Verification items for this drawing (mm, ordinates from the low corner). A direction names the side the tool comes from. Round coordinates to 2 decimals unless told otherwise and drop trailing zeros. Loops run counter-clockwise (first coordinate to the right, second up) from the corner with the lowest first, then second, coordinate; pieces in that order, holes last. Notation, with made-up numbers: M -16.75,20 L 31.25,20 A38 ccw 31.25,59 Z; hole C 84.5,38.25 d4. An arc over 180 degrees is marked long. Write item = value, one per line. Start each with the question number.
(1) Cross-section at D-D on x = 5.1. Record the boundary of the cut face in (y, z), plus the area to 3 significant figures.
(2) Cross-section at C-C on y = 11.25. Record the boundary of the cut face in (x, z), plus the area to 3 significant figures.
(3) Scan lines: L1, parallel to Y at x = 4.8, z = 4.45; L2, parallel to Z at x = 2.85, y = 4.5; L3, parallel to X at y = 5.25, z = 3.9. Record each from-to range of solid material in increasing order. Write a range as from..to.
(4) Go/stop test with flat-tipped pins: P1, Ø1.5, axis at x = 4.5, z = 1.5, coming from the -Y side; P2, Ø1.5, axis at y = 5, z = 5, coming from the -X side (1 decimal); P3, Ø3.5, axis at y = 5, z = 3, coming from the +X side. Record where each tip stops, or that it passes through.
(5) Cross-section at B-B on z = 2. Record the boundary of the cut face in (x, y), plus the area to 3 significant figures.
(6) Set-up check for the marked faces 1, 2, 3, 4 and 5: record each of +Z, -Z, +X, -X, +Y, -Y from which the full face is reachable in a straight line by a thin tool's end or side.
(7) Cross-section at A-A on x = 0.45. Record the boundary of the cut face in (y, z).
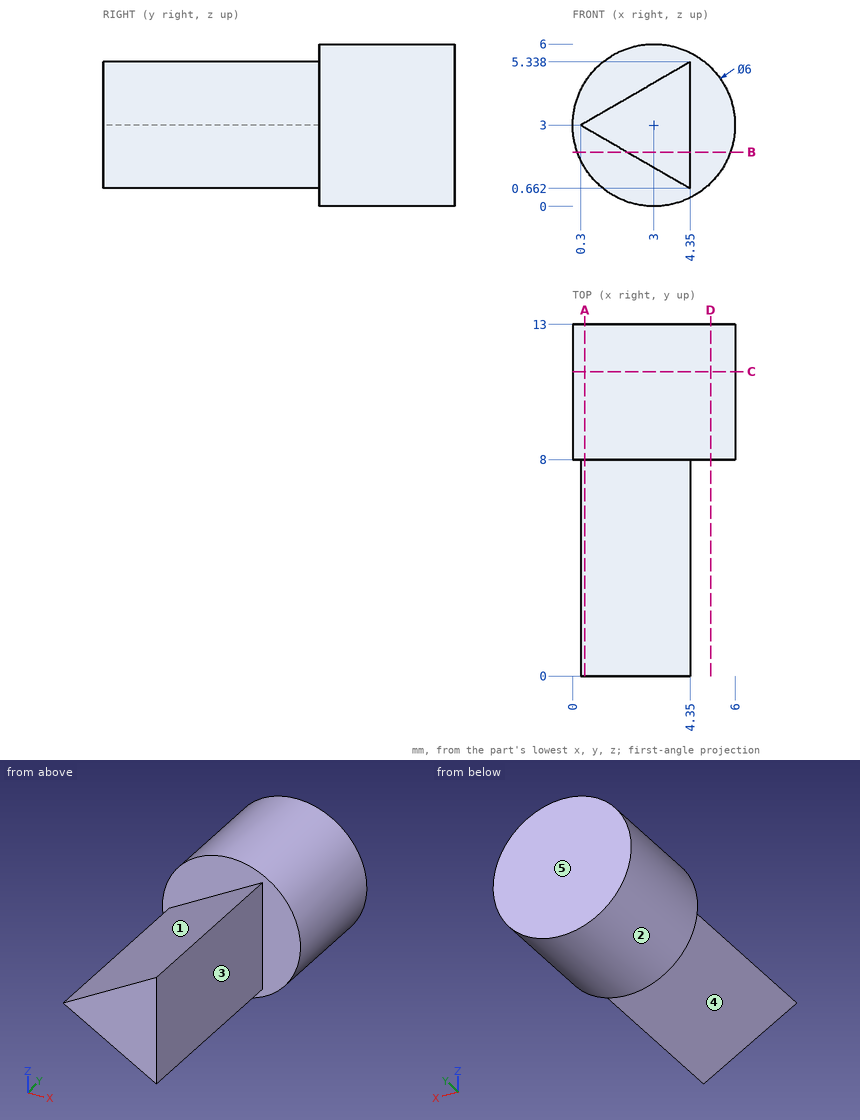
Result:
q1.outline = M 8,0.86 L 13,0.86 L 13,5.14 L 8,5.14 Z
q1.area = 21.4 mm^2
q2.outline = C 3,3 d6
q2.area = 28.3 mm^2
q3.L1 = 8..13
q3.L2 = 1.53..4.47
q3.L3 = 1.86..4.35
q4.P1 = 0
q4.P2 = 2.5
q4.P3 = 4.35
q5.outline = M 0.17,8 L 2.03,8 L 2.03,0 L 4.35,0 L 4.35,8 L 5.83,8 L 5.83,13 L 0.17,13 Z
q5.area = 46.8 mm^2
q6.face_1 = +Z, -X, -Y
q6.face_2 = +Y, -Y
q6.face_3 = +Z, -Z, +X, -Y
q6.face_4 = -Z, -X, -Y
q6.face_5 = +Z, -Z, +X, -X, +Y
q7.outline = M 0,2.91 L 8,2.91 L 8,1.42 L 13,1.42 L 13,4.58 L 8,4.58 L 8,3.09 L 0,3.09 Z
